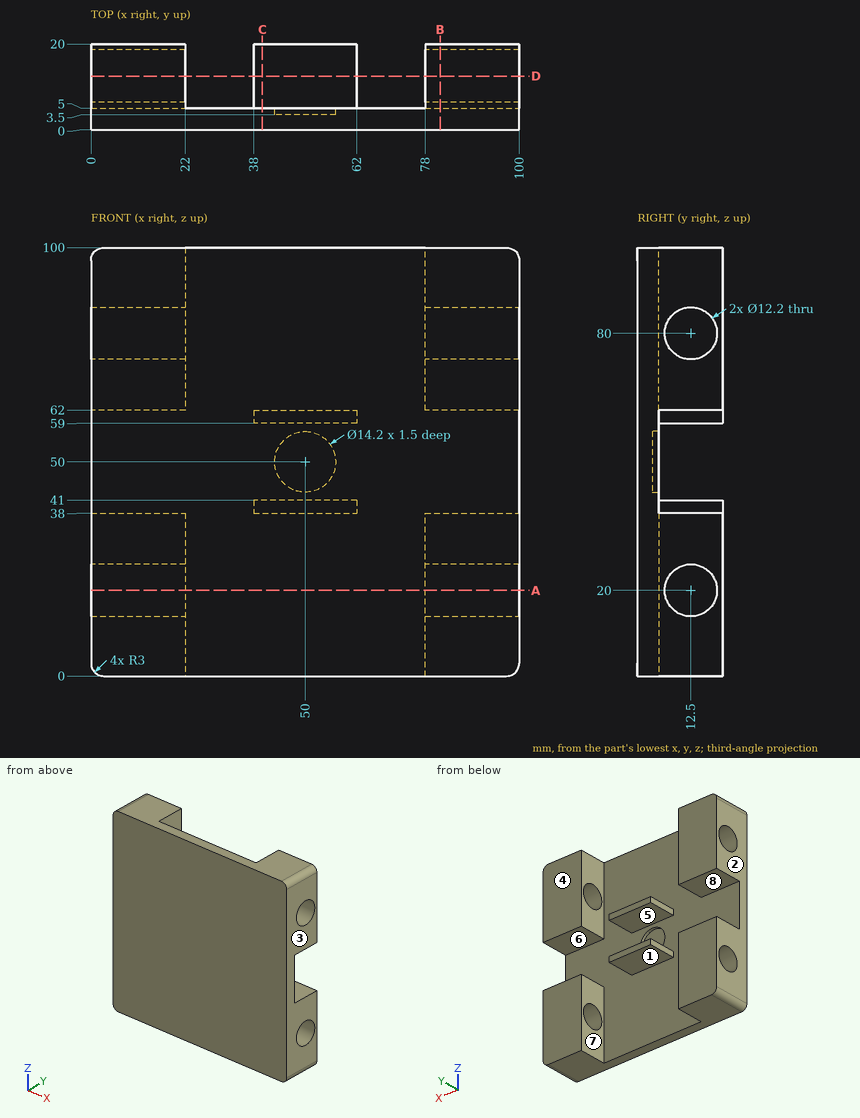
Can you work these out from the drawing? Everything is in mm from the part's minimum corner. A direction names the side the tool comes from. Round coordinates to 2 decimals unless told otherwise and drop trailing zeros. Write each loop counter-clockwise with the first axis right and the second up, starting at its lowest first coordinate (ties: lowest second). Pieces come first, ordered by that corner, then holes.
1. Suppose I cut it at A-A (z = 20). List the corners of the cut face in (x, y) for me, and give its area (3 significant figures).
2. Suppose I cut it at D-D (y = 12.5). State how many separate pieces and enclosed holes the cut face has, and give its area (3 significant figures).
3. Will these pins go through, and if not, where does the flat tip stop? pin 1 Ø7.5 at (y, z) = (14.5, 19.5) entering from +X; pin 2 Ø2.5 at (y, z) = (12, 39.5) entering from -X; pin 3 Ø7.5 at (x, y) = (50, 13) entering from -Z; pin 4 Ø7.5 at (x, y) = (54, 10) entering from +Z.
4. I need wall thicknesses on L1, parallel to Z at x = 14, y = 12; L2, parallel to Y at x = 13, z = 20; L3, parallel to X at y = 19, z = 13. Which ranges of each line are inside material? Lowest first, please.
5. If we mould it in two halves opening along X, with no side actions, what happens to the marked faces 1, 2, 3 and 4? For each: released by +X, released by -X, zero draft, split by the parting line, or undercut.
6. Suppose I cut it at C-C (x = 40). List the corners of the cut face in (y, z) for me, and give its area (3 significant figures).
7. Suppose I cut it at B-B (x = 81.5). List the corners of the cut face in (y, z) for me, and give its area (3 significant figures).
8. For the marked faces 5, 6, 7 and 8, which set-ups out of +Z, -Z, +X, -X, +Y, -Y let a thin tool reach every point of the face, with its end or its side?
Answer sheet:
1. outline: (0, 0) - (100, 0) - (100, 6.4) - (78, 6.4) - (78, 5) - (22, 5) - (22, 6.4) - (0, 6.4) - close; (0, 18.6) - (22, 18.6) - (22, 20) - (0, 20) - close; (78, 18.6) - (100, 18.6) - (100, 20) - (78, 20) - close
1. area: 623 mm2
2. separate pieces: 10
2. enclosed holes: 0
2. area: 2,410 mm2
3. pin 1: passes through
3. pin 2: stops at x = 38
3. pin 3: stops at z = 38
3. pin 4: stops at z = 62
4. L1: z = 0 to 13.92, 26.08 to 38, 62 to 73.92, 86.08 to 100
4. L2: y = 0 to 6.4, 18.6 to 20
4. L3: x = 0 to 22, 78 to 100
5. face 1: undercut
5. face 2: released by -X
5. face 3: released by +X
5. face 4: zero draft
6. outline: (0, 0) - (5, 0) - (5, 38) - (20, 38) - (20, 41) - (5, 41) - (5, 59) - (20, 59) - (20, 62) - (5, 62) - (5, 100) - (0, 100) - close
6. area: 590 mm2
7. outline: (0, 0) - (20, 0) - (20, 38) - (5, 38) - (5, 62) - (20, 62) - (20, 100) - (0, 100) - close; hole circle Ø12.2 at (12.5, 20); hole circle Ø12.2 at (12.5, 80)
7. area: 1,410 mm2
8. face 5: +X, -X, +Y
8. face 6: +X, +Y
8. face 7: +Z, -Z, +Y
8. face 8: -X, +Y
